Could you check a few things on this model? Use its own coordinates, in mm. A direction names the side the tool comes from. Give positions to 0.01 mm unless a question says otherwise; leave off trailing zeros. Loops run counter-clockwise (first coordinate to the right, second up) from the corner with the lowest first, then second, coordinate; pieces in that order, holes last.
1. I need wall thicknesses on line 1 along Z through (x, y) = (-19, 2.6); line 2 along Z through (x, y) = (12.5, 2.85); line 3 along X through (y, z) = (3.5, -48.5). Which ranges of each line are inside material? Lowest first, please.
2. For faces 1 (the flat face through (-21, 3, -58)), 2 (the flat face through (29, 3, -30)), 3 (the flat face through (-15, 3, 58)), 4 (the flat face through (-22, 3, 47)), which set-ups out of +Z, -Z, +X, -X, +Y, -Y let a thin tool reach every point of the face, with its end or its side?
3. Imagine slicing it at B-B (z = -13.5). List the corners of the cut face in (x, y) for me, plus the area to 4 significant figures.
4. Imagine slicing it at A-A (y = 3.5). Count the separate pieces of the cut face and the enclosed holes in it, plus the area to 3 significant figures.
5. Thinking about a two-plate mould opening in X: for faces 5 (the flat face through (0, 0, 1)), 6 (the flat face through (32, 3, 0)), 7 (the flat face through (-10, 3, 47)), which applies, +X half, -X half, draft (parallel to the pull), parting line (faces both ways), or undercut?
6. For P1, Ø3, axis at y = 2.5, z = 15.5, coming from the -X side; P2, Ø1.6, axis at x = 17.5, y = 1.5, coming from the +Z side; P3, Ø3, axis at x = 18.5, y = 2.5, coming from the -Z side, each with a flat end and sliding along its axis, tell me the tip position at first contact or that it passes through.
Autodesk Inventor part; units mm, degrees
ref_plane "YZ Plane" through (0, 0, 0) normal (1, 0, 0) x (0, 1, 0)
ref_plane "XZ Plane" through (0, 0, 0) normal (0, 1, 0) x (-1, 0, 0)
ref_plane "XY Plane" through (0, 0, 0) normal (0, 0, 1) x (1, 0, 0)
sketch "Block1" plane through (0, 0, 0) normal (0, 0, 1) x (1, 0, 0)
  line L0 (-15.1, 61.1) -> (15.1, 61.1)
  line L1 (15.1, 61.1) -> (15.1, 52.1)
  line L2 (15.1, 52.1) -> (20.9, 52.1)
  line L3 (20.9, 52.1) -> (20.9, 61.1)
  line L4 (20.9, 61.1) -> (35.6, 61.1)
  line L5 (35.6, 61.1) -> (35.6, 29.9)
  line L6 (35.6, 29.9) -> (26.6, 29.9)
  line L7 (26.6, 29.9) -> (26.6, 10.1)
  line L8 (26.6, 10.1) -> (35.6, 10.1)
  line L9 (35.6, 10.1) -> (35.6, -10.1)
  line L10 (35.6, -10.1) -> (26.6, -10.1)
  line L11 (26.6, -10.1) -> (26.6, -29.9)
  line L12 (26.6, -29.9) -> (35.6, -29.9)
  line L13 (35.6, -29.9) -> (35.6, -61.1)
  line L14 (35.6, -61.1) -> (20.9, -61.1)
  line L15 (20.9, -61.1) -> (20.9, -52.1)
  line L16 (20.9, -52.1) -> (15.1, -52.1)
  line L17 (15.1, -52.1) -> (15.1, -61.1)
  line L18 (15.1, -61.1) -> (-15.1, -61.1)
  line L19 (-15.1, -61.1) -> (-15.1, -52.1)
  line L20 (-15.1, -52.1) -> (-20.9, -52.1)
  line L21 (-20.9, -52.1) -> (-20.9, -61.1)
  line L22 (-20.9, -61.1) -> (-35.6, -61.1)
  line L23 (-35.6, -61.1) -> (-35.6, -29.9)
  line L24 (-35.6, -29.9) -> (-26.6, -29.9)
  line L25 (-26.6, -29.9) -> (-26.6, -10.1)
  line L26 (-26.6, -10.1) -> (-35.6, -10.1)
  line L27 (-35.6, -10.1) -> (-35.6, 10.1)
  line L28 (-35.6, 10.1) -> (-26.6, 10.1)
  line L29 (-26.6, 10.1) -> (-26.6, 29.9)
  line L30 (-26.6, 29.9) -> (-35.6, 29.9)
  line L31 (-35.6, 29.9) -> (-35.6, 61.1)
  line L32 (-35.6, 61.1) -> (-20.9, 61.1)
  line L33 (-20.9, 61.1) -> (-20.9, 52.1)
  line L34 (-20.9, 52.1) -> (-15.1, 52.1)
  line L35 (-15.1, 52.1) -> (-15.1, 61.1)
  line L36 (-9.9, 50.1) -> (-22.1, 50.1)
  line L37 (-22.1, 50.1) -> (-22.1, 40.9)
  line L38 (-22.1, 40.9) -> (-9.9, 40.9)
  line L39 (-9.9, 40.9) -> (-9.9, 50.1)
  line L40 (22.1, 50.1) -> (22.1, 40.9)
  line L41 (22.1, 40.9) -> (9.9, 40.9)
  line L42 (9.9, 40.9) -> (9.9, 50.1)
  line L43 (9.9, 50.1) -> (22.1, 50.1)
  line L44 (22.1, -40.9) -> (9.9, -40.9)
  line L45 (9.9, -40.9) -> (9.9, -50.1)
  line L46 (9.9, -50.1) -> (22.1, -50.1)
  line L47 (22.1, -50.1) -> (22.1, -40.9)
  line L48 (-9.9, -40.9) -> (-22.1, -40.9)
  line L49 (-22.1, -40.9) -> (-22.1, -50.1)
  line L50 (-22.1, -50.1) -> (-9.9, -50.1)
  line L51 (-9.9, -50.1) -> (-9.9, -40.9)
  point P0 (0, 0)
sketch "Block2" plane through (0, 0, 0) normal (0, 0, 1) x (1, 0, 0)
  line L0 (20.8, 61.2) -> (35.7, 61.2)
  line L1 (35.7, 61.2) -> (35.7, 29.8)
  line L2 (35.7, 29.8) -> (26.7, 29.8)
  line L3 (26.7, 29.8) -> (26.7, 10.2)
  line L4 (26.7, 10.2) -> (35.7, 10.2)
  line L5 (35.7, 10.2) -> (35.7, -10.2)
  line L6 (35.7, -10.2) -> (26.7, -10.2)
  line L7 (26.7, -10.2) -> (26.7, -29.8)
  line L8 (26.7, -29.8) -> (35.7, -29.8)
  line L9 (35.7, -29.8) -> (35.7, -61.2)
  line L10 (35.7, -61.2) -> (20.8, -61.2)
  line L11 (20.8, -61.2) -> (20.8, -52.2)
  line L12 (20.8, -52.2) -> (15.2, -52.2)
  line L13 (15.2, -52.2) -> (15.2, -61.2)
  line L14 (15.2, -61.2) -> (-15.2, -61.2)
  line L15 (-15.2, -61.2) -> (-15.2, -52.2)
  line L16 (-15.2, -52.2) -> (-20.8, -52.2)
  line L17 (-20.8, -52.2) -> (-20.8, -61.2)
  line L18 (-20.8, -61.2) -> (-35.7, -61.2)
  line L19 (-35.7, -61.2) -> (-35.7, -29.8)
  line L20 (-35.7, -29.8) -> (-26.7, -29.8)
  line L21 (-26.7, -29.8) -> (-26.7, -10.2)
  line L22 (-26.7, -10.2) -> (-35.7, -10.2)
  line L23 (-35.7, -10.2) -> (-35.7, 10.2)
  line L24 (-35.7, 10.2) -> (-26.7, 10.2)
  line L25 (-26.7, 10.2) -> (-26.7, 29.8)
  line L26 (-26.7, 29.8) -> (-35.7, 29.8)
  line L27 (-35.7, 29.8) -> (-35.7, 61.2)
  line L28 (-35.7, 61.2) -> (-20.8, 61.2)
  line L29 (-20.8, 61.2) -> (-20.8, 52.2)
  line L30 (-20.8, 52.2) -> (-15.2, 52.2)
  line L31 (-15.2, 52.2) -> (-15.2, 61.2)
  line L32 (-15.2, 61.2) -> (15.2, 61.2)
  line L33 (15.2, 61.2) -> (15.2, 52.2)
  line L34 (15.2, 52.2) -> (20.8, 52.2)
  line L35 (20.8, 52.2) -> (20.8, 61.2)
  line L36 (22.2, 50.2) -> (22.2, 40.8)
  line L37 (22.2, 40.8) -> (9.8, 40.8)
  line L38 (9.8, 40.8) -> (9.8, 50.2)
  line L39 (9.8, 50.2) -> (22.2, 50.2)
  line L40 (-9.8, 50.2) -> (-22.2, 50.2)
  line L41 (-22.2, 50.2) -> (-22.2, 40.8)
  line L42 (-22.2, 40.8) -> (-9.8, 40.8)
  line L43 (-9.8, 40.8) -> (-9.8, 50.2)
  line L44 (-9.8, -40.8) -> (-22.2, -40.8)
  line L45 (-22.2, -40.8) -> (-22.2, -50.2)
  line L46 (-22.2, -50.2) -> (-9.8, -50.2)
  line L47 (-9.8, -50.2) -> (-9.8, -40.8)
  line L48 (22.2, -40.8) -> (9.8, -40.8)
  line L49 (9.8, -40.8) -> (9.8, -50.2)
  line L50 (9.8, -50.2) -> (22.2, -50.2)
  line L51 (22.2, -50.2) -> (22.2, -40.8)
  point P0 (0, 0)
sketch "Block3" plane through (0, 0, 0) normal (0, 0, 1) x (1, 0, 0)
  line L0 (20.9, 61.1) -> (35.6, 61.1)
  line L1 (35.6, 61.1) -> (35.6, 29.9)
  line L2 (35.6, 29.9) -> (26.6, 29.9)
  line L3 (26.6, 29.9) -> (26.6, 10.1)
  line L4 (26.6, 10.1) -> (35.6, 10.1)
  line L5 (35.6, 10.1) -> (35.6, -10.1)
  line L6 (35.6, -10.1) -> (26.6, -10.1)
  line L7 (26.6, -10.1) -> (26.6, -29.9)
  line L8 (26.6, -29.9) -> (35.6, -29.9)
  line L9 (35.6, -29.9) -> (35.6, -61.1)
  line L10 (35.6, -61.1) -> (20.9, -61.1)
  line L11 (20.9, -61.1) -> (20.9, -52.1)
  line L12 (20.9, -52.1) -> (15.1, -52.1)
  line L13 (15.1, -52.1) -> (15.1, -61.1)
  line L14 (15.1, -61.1) -> (-15.1, -61.1)
  line L15 (-15.1, -61.1) -> (-15.1, -52.1)
  line L16 (-15.1, -52.1) -> (-20.9, -52.1)
  line L17 (-20.9, -52.1) -> (-20.9, -61.1)
  line L18 (-20.9, -61.1) -> (-35.6, -61.1)
  line L19 (-35.6, -61.1) -> (-35.6, -29.9)
  line L20 (-35.6, -29.9) -> (-26.6, -29.9)
  line L21 (-26.6, -29.9) -> (-26.6, -10.1)
  line L22 (-26.6, -10.1) -> (-35.6, -10.1)
  line L23 (-35.6, -10.1) -> (-35.6, 10.1)
  line L24 (-35.6, 10.1) -> (-26.6, 10.1)
  line L25 (-26.6, 10.1) -> (-26.6, 29.9)
  line L26 (-26.6, 29.9) -> (-35.6, 29.9)
  line L27 (-35.6, 29.9) -> (-35.6, 61.1)
  line L28 (-35.6, 61.1) -> (-20.9, 61.1)
  line L29 (-20.9, 61.1) -> (-20.9, 52.1)
  line L30 (-20.9, 52.1) -> (-15.1, 52.1)
  line L31 (-15.1, 52.1) -> (-15.1, 61.1)
  line L32 (-15.1, 61.1) -> (15.1, 61.1)
  line L33 (15.1, 61.1) -> (15.1, 52.1)
  line L34 (15.1, 52.1) -> (20.9, 52.1)
  line L35 (20.9, 52.1) -> (20.9, 61.1)
  line L36 (22.1, 50.1) -> (22.1, 40.9)
  line L37 (22.1, 40.9) -> (9.9, 40.9)
  line L38 (9.9, 40.9) -> (9.9, 50.1)
  line L39 (9.9, 50.1) -> (22.1, 50.1)
  line L40 (-9.9, 50.1) -> (-22.1, 50.1)
  line L41 (-22.1, 50.1) -> (-22.1, 40.9)
  line L42 (-22.1, 40.9) -> (-9.9, 40.9)
  line L43 (-9.9, 40.9) -> (-9.9, 50.1)
  line L44 (-9.9, -40.9) -> (-22.1, -40.9)
  line L45 (-22.1, -40.9) -> (-22.1, -50.1)
  line L46 (-22.1, -50.1) -> (-9.9, -50.1)
  line L47 (-9.9, -50.1) -> (-9.9, -40.9)
  line L48 (22.1, -40.9) -> (9.9, -40.9)
  line L49 (9.9, -40.9) -> (9.9, -50.1)
  line L50 (9.9, -50.1) -> (22.1, -50.1)
  line L51 (22.1, -50.1) -> (22.1, -40.9)
  point P0 (0, 0)
sketch "Block4" plane through (0, 0, 0) normal (0, 0, 1) x (1, 0, 0)
  line L0 (-15.08, 61.08) -> (15.08, 61.08)
  line L1 (15.08, 61.08) -> (15.08, 55.58)
  line L2 (15.08, 55.58) -> (20.92, 55.58)
  line L3 (20.92, 55.58) -> (20.92, 61.08)
  line L4 (20.92, 61.08) -> (32.08, 61.08)
  line L5 (32.08, 61.08) -> (32.08, 29.92)
  line L6 (32.08, 29.92) -> (26.58, 29.92)
  line L7 (26.58, 29.92) -> (26.58, 10.08)
  line L8 (26.58, 10.08) -> (32.08, 10.08)
  line L9 (32.08, 10.08) -> (32.08, -10.08)
  line L10 (32.08, -10.08) -> (26.58, -10.08)
  line L11 (26.58, -10.08) -> (26.58, -29.92)
  line L12 (26.58, -29.92) -> (32.08, -29.92)
  line L13 (32.08, -29.92) -> (32.08, -61.08)
  line L14 (32.08, -61.08) -> (20.92, -61.08)
  line L15 (20.92, -61.08) -> (20.92, -55.58)
  line L16 (20.92, -55.58) -> (15.08, -55.58)
  line L17 (15.08, -55.58) -> (15.08, -61.08)
  line L18 (15.08, -61.08) -> (-15.08, -61.08)
  line L19 (-15.08, -61.08) -> (-15.08, -55.58)
  line L20 (-15.08, -55.58) -> (-20.92, -55.58)
  line L21 (-20.92, -55.58) -> (-20.92, -61.08)
  line L22 (-20.92, -61.08) -> (-32.08, -61.08)
  line L23 (-32.08, -61.08) -> (-32.08, -29.92)
  line L24 (-32.08, -29.92) -> (-26.58, -29.92)
  line L25 (-26.58, -29.92) -> (-26.58, -10.08)
  line L26 (-26.58, -10.08) -> (-32.08, -10.08)
  line L27 (-32.08, -10.08) -> (-32.08, 10.08)
  line L28 (-32.08, 10.08) -> (-26.58, 10.08)
  line L29 (-26.58, 10.08) -> (-26.58, 29.92)
  line L30 (-26.58, 29.92) -> (-32.08, 29.92)
  line L31 (-32.08, 29.92) -> (-32.08, 61.08)
  line L32 (-32.08, 61.08) -> (-20.92, 61.08)
  line L33 (-20.92, 61.08) -> (-20.92, 55.58)
  line L34 (-20.92, 55.58) -> (-15.08, 55.58)
  line L35 (-15.08, 55.58) -> (-15.08, 61.08)
  line L36 (-9.92, 50.08) -> (-22.08, 50.08)
  line L37 (-22.08, 50.08) -> (-22.08, 44.42)
  line L38 (-22.08, 44.42) -> (-9.92, 44.42)
  line L39 (-9.92, 44.42) -> (-9.92, 50.08)
  line L40 (22.08, 50.08) -> (22.08, 44.42)
  line L41 (22.08, 44.42) -> (9.92, 44.42)
  line L42 (9.92, 44.42) -> (9.92, 50.08)
  line L43 (9.92, 50.08) -> (22.08, 50.08)
  line L44 (-9.92, -44.42) -> (-22.08, -44.42)
  line L45 (-22.08, -44.42) -> (-22.08, -50.08)
  line L46 (-22.08, -50.08) -> (-9.92, -50.08)
  line L47 (-9.92, -50.08) -> (-9.92, -44.42)
  line L48 (22.08, -44.42) -> (9.92, -44.42)
  line L49 (9.92, -44.42) -> (9.92, -50.08)
  line L50 (9.92, -50.08) -> (22.08, -50.08)
  line L51 (22.08, -50.08) -> (22.08, -44.42)
  point P0 (0, 0)
sketch "Sketch1" plane through (0, 0, 0) normal (0, 1, 0) x (-1, 0, 0)
  line L0 (32, -50) -> (-32, -50)
  line L1 (-32, -50) -> (-32, 50)
  line L2 (-32, 50) -> (32, 50)
  line L3 (32, 50) -> (32, -50)
  line L4 (32, -50) -> (-32, 50) construction
  line L5 (-32, -50) -> (32, 50) construction
  point P0 (0, 0)
  dimension "d0" = 64
  dimension "d1" = 100
extrude "Extrusion1" add sketch "Sketch1" along normal blind 5.5
sketch "Sketch5" plane through (0, 5.5, 0) normal (0, 1, 0) x (1, 0, 0)
  line L0 (32, 50) -> (-32, 50)
  line L1 (-32, 50) -> (-32, -50)
  line L2 (-32, 30) -> (-26.5, 30)
  line L3 (-26.5, 30) -> (-26.5, 10)
  line L4 (-26.5, 10) -> (-32, 10)
  line L5 (-32, 10) -> (-32, 30)
  line L6 (-66.327, 0) -> (148.7623, 0)
  line L7 (0, 85.6282) -> (0, -86.069)
  line L8 (-32, -30) -> (-26.5, -30)
  line L9 (-26.5, -30) -> (-26.5, -10)
  line L10 (-26.5, -10) -> (-32, -10)
  line L11 (-32, -10) -> (-32, -30)
  line L12 (32, 30) -> (26.5, 30)
  line L13 (26.5, 30) -> (26.5, 10)
  line L14 (26.5, 10) -> (32, 10)
  line L15 (32, 10) -> (32, 30)
  line L16 (32, -30) -> (26.5, -30)
  line L17 (26.5, -30) -> (26.5, -10)
  line L18 (26.5, -10) -> (32, -10)
  line L19 (32, -10) -> (32, -30)
  point P0 (0, 0)
  dimension "d12" = 20
  dimension "d13" = 20
  dimension "d14" = 5.5
extrude "Extrusion3" cut sketch "Sketch5" against normal through all contours L10 L9 L8 L1 | L2 L3 L4 L1 | L15 L14 L13 L12 | L16 L17 L18 L19
sketch "Sketch6" plane through (0, 5.5, 0) normal (0, 1, 0) x (1, 0, 0)
  line L0 (32, 50) -> (-32, 50)
  line L1 (-66.327, 0) -> (148.7623, 0)
  line L2 (0, 85.6282) -> (0, -86.069)
  line L3 (-22, 50) -> (-10, 50)
  line L4 (-10, 50) -> (-10, 44.5)
  line L5 (-10, 44.5) -> (-22, 44.5)
  line L6 (-22, 44.5) -> (-22, 50)
  line L7 (22, 50) -> (10, 50)
  line L8 (10, 50) -> (10, 44.5)
  line L9 (10, 44.5) -> (22, 44.5)
  line L10 (22, 44.5) -> (22, 50)
  line L11 (-22, -50) -> (-10, -50)
  line L12 (-10, -50) -> (-10, -44.5)
  line L13 (-10, -44.5) -> (-22, -44.5)
  line L14 (-22, -44.5) -> (-22, -50)
  line L15 (10, -44.5) -> (22, -44.5)
  line L16 (22, -50) -> (10, -50)
  line L17 (10, -50) -> (10, -44.5)
  line L18 (22, -44.5) -> (22, -50)
  point P0 (0, 0)
  dimension "d17" = 5.5
  dimension "d18" = 12
  dimension "d19" = 20
extrude "Extrusion4" cut sketch "Sketch6" against normal through all
sketch "Sketch7" plane through (0, 0, 0) normal (0, -1, 0) x (1, 0, 0)
  line L0 (-32, -50) -> (32, -50)
  line L1 (32, -50) -> (32, -61)
  line L2 (32, -61) -> (-32, -61)
  line L3 (-32, -61) -> (-32, -50)
  line L4 (-66.327, 0) -> (148.7623, 0)
  line L5 (0, -85.6282) -> (0, 86.069)
  line L6 (-15, -61) -> (-21, -61)
  line L7 (-21, -61) -> (-21, -55.5)
  line L8 (-21, -55.5) -> (-15, -55.5)
  line L9 (-15, -55.5) -> (-15, -61)
  line L10 (15, -61) -> (21, -61)
  line L11 (21, -61) -> (21, -55.5)
  line L12 (21, -55.5) -> (15, -55.5)
  line L13 (15, -55.5) -> (15, -61)
  line L14 (-32, 50) -> (32, 50)
  line L15 (32, 50) -> (32, 61)
  line L16 (32, 61) -> (-32, 61)
  line L17 (-32, 61) -> (-32, 50)
  line L18 (-32, 50) -> (-22, 50)
  line L19 (-10, 50) -> (10, 50)
  line L20 (22, 50) -> (32, 50)
  line L21 (-15, 61) -> (-21, 61)
  line L22 (-21, 61) -> (-21, 55.5)
  line L23 (-21, 55.5) -> (-15, 55.5)
  line L24 (-15, 55.5) -> (-15, 61)
  line L25 (21, 55.5) -> (15, 55.5)
  line L26 (15, 55.5) -> (15, 61)
  line L27 (15, 61) -> (21, 61)
  line L28 (21, 61) -> (21, 55.5)
  point P0 (0, 0)
  point P1 (32, -50)
  dimension "d22" = 11
  dimension "d23" = 6
  dimension "d24" = 5.5
  dimension "d32" = 15
  dimension "d55" = 64
extrude "Extrusion7" add sketch "Sketch7" against normal blind 5.5 contours L14 L17 L16 L22 L23 L24 L5 | L5 L16 L26 L25 L28 L15 L14 | L0 L5 L2 L9 L8 L7 L3 | L0 L1 L2 L11 L12 L13 L5
equation "\"d2\" = Wt"
equation "\"d14\" = Wt"
equation "\"d15\" = Wt"
equation "\"d17\" = Wt"
equation "\"d20\" = Wt"
equation "\"d24\" = Wt"
equation "\"d55\" = d0"
equation "\"d33\" = Wt"
properties part number "holder_ceil_plate" material "Wood (Birch)"
Derived:
1. line 1: z = -55.5 to -50, -44.5 to 44.5, 50 to 55.5
1. line 2: z = -61 to -50, -44.5 to 44.5, 50 to 61
1. line 3: x = -32 to -22, -10 to 10, 22 to 32
2. face 1: -Z, +Y, -Y
2. face 2: +X, +Y, -Y
2. face 3: +Z, +Y, -Y
2. face 4: +Y, -Y
3. outline: (-26.5, 0) - (26.5, 0) - (26.5, 5.5) - (-26.5, 5.5) - close
3. area: 291.5 mm2
4. separate pieces: 1
4. enclosed holes: 4
4. area: 6,970 mm2
5. face 5: draft
5. face 6: +X half
5. face 7: undercut
6. P1: stops at x = -26.5
6. P2: stops at z = 55.5
6. P3: stops at z = -55.5
